Input: part model. Units: mm. Frame: model coordinates. A direction names the side the tool comes from. Coordinates: 2 decimals unless noted, no trailing zeros. Write each loop counter-clockwise with the first axis right and the second up, starting at its lowest first coordinate (ties: lowest second). Pieces come first, ordered by that corner, then holes. Notation, with made-up numbers: (27, 71.5) - (59, 71.5) arc R11 ccw to (59, 79.5) - close; hole circle Ø9 at (-18, 58.25). An arc over 180 degrees is marked (long way). Put each result on its own line as item: value. Start each with the question number.
1. Pull-direction query (Y, two-part tool) for faces 4 (the cylindrical face through (-715.32, 1615.44, -223.05)), 5 (the cylindrical face through (-652.31, 1811.02, -88.74)), 6 (the flat face through (-678, 1443, -180)); classes: released by +Y, released by -Y, zero draft, split by the parting line, or undercut.
2. Cut plane C-C, the plane x = -686. Return loops of the section in (y, z), and give its area (3 significant figures).
3. Cut plane A-A, the plane y = 1465. Return loops of the section in (x, z).
4. Access query for faces 1 (the cylindrical face through (-791.677, 1870.362, -250.236)), 2 (the flat face through (-678, 1443, -330)), 3 (the cylindrical face through (-625.073, 1799.298, -258.88)). Directions: +Z, -Z, +X, -X, +Y, -Y. A direction counts if a zero-diameter tool reaches every point of the face in a straight line with its end or side. Return the directions, or none.
5. Cut plane B-B, the plane z = -314. Return loops of the section in (x, y), and give its area (3 significant figures).
6. Line query: line 1 (Y direction, x = -700, z = -309.5); line 2 (Y direction, x = -700, z = -237); line 3 (Z direction, x = -730.5, y = 1462.5). Output: solid intervals per line, ascending.
7. Cut plane D-D, the plane y = 1796. Return loops of the section in (x, z), and give its area (3 significant figures).
8. Pin query (flat end, axial travel): pin 1 (1 mm diameter, centred on x = -741.5, z = -78, fed in from -Y); pin 2 (1 mm diameter, centred on x = -722.5, y = 1699.5, fed in from -Z); pin 3 (8 mm diameter, centred on x = -757, z = -238.5, fed in from -Y); pin 4 (1.5 mm diameter, centred on y = 1483, z = -177.5, fed in from -X). Return the tip coordinate at first contact, or that it passes through.
from build123d import *

# Parameters (mm, degrees)
SKETCH1_R           = 50
BOSS_EXTRUDE1_DEPTH = 180
SKETCH2_R           = 75
BOSS_EXTRUDE2_DEPTH = 160
SKETCH3_R           = 75
BOSS_EXTRUDE3_DEPTH = 128.18
SKETCH4_R           = 40
BOSS_EXTRUDE4_DEPTH = 300
SKETCH5_R           = 50
SKETCH5_R_2         = 30
BOSS_EXTRUDE5_DEPTH = 150


with BuildPart() as part:
    # Sketch1 → Boss-Extrude1 (new body)
    with BuildSketch(Plane.XY):
        with Locations((-700, 1796)):
            Circle(SKETCH1_R)
    extrude(amount=-BOSS_EXTRUDE1_DEPTH)

    # Sketch2 → Boss-Extrude2 (add)
    with BuildSketch(Plane(origin=(0, 0, -180), x_dir=(-1, 0, 0), z_dir=(0, 0, -1))):
        with Locations((700, 1796)):
            Circle(SKETCH2_R)
    extrude(amount=BOSS_EXTRUDE2_DEPTH)

    # Sketch3 → Boss-Extrude3 (add)
    with BuildSketch(Plane(origin=(-700, 0, 0), x_dir=(0, 0, -1), z_dir=(1, 0, 0))):
        with Locations((260, 1796)):
            Circle(SKETCH3_R)
    extrude(amount=-BOSS_EXTRUDE3_DEPTH)

    # Sketch4 → Boss-Extrude4 (add)
    with BuildSketch(Plane(origin=(0, 1795, 0), x_dir=(-1, 0, 0), z_dir=(0, 1, 0))):
        with Locations(Location((700, -260, 0), (0, 0, 90))):
            Circle(SKETCH4_R)
    extrude(amount=-BOSS_EXTRUDE4_DEPTH)

    # Sketch5 → Boss-Extrude5 (add)
    with BuildSketch(Plane.XY.offset(-180)):
        with Locations((-700, 1465)):
            Circle(SKETCH5_R)
        with Locations((-700, 1465)):
            Circle(SKETCH5_R_2, mode=Mode.SUBTRACT)
    extrude(amount=-BOSS_EXTRUDE5_DEPTH)


solid = part.part
Report:
1. face 4: undercut
1. face 5: split by the parting line
1. face 6: zero draft
2. outline: (1417, -330) - (1438.47, -330) - (1438.47, -180) - (1417, -180) - close; (1491.53, -330) - (1513, -330) - (1513, -297.47) - (1722.32, -297.47) - (1722.32, -340) - (1869.68, -340) - (1869.68, -180) - (1844, -180) - (1844, 0) - (1748, 0) - (1748, -180) - (1722.32, -180) - (1722.32, -222.53) - (1513, -222.53) - (1513, -180) - (1491.53, -180) - close
2. area: 63,000 mm^2
3. outline: (-750, -330) - (-730, -330) - (-730, -180) - (-750, -180) - close; (-670, -330) - (-650, -330) - (-650, -180) - (-670, -180) - close
4. face 1: -X
4. face 2: -Z, +X, -X, -Y
4. face 3: none
5. outline: (-828.18, 1743.95) - (-754, 1743.95) arc R75 ccw (long way) to (-754, 1848.05) - (-828.18, 1848.05) - close; circle Ø100 at (-700, 1465); hole circle Ø60 at (-700, 1465)
5. area: 28,900 mm^2
6. line 1: y = 1415 to 1435, 1495 to 1515, 1721 to 1871
6. line 2: y = 1415 to 1435, 1495 to 1871
6. line 3: z = -330 to -180
7. outline: (-828.18, -335) - (-775, -335) - (-775, -340) - (-625, -340) - (-625, -180) - (-650, -180) - (-650, 0) - (-750, 0) - (-750, -180) - (-775, -180) - (-775, -185) - (-828.18, -185) - close
7. area: 50,000 mm^2
8. pin 1: stops at y = 1767.38
8. pin 2: stops at z = -293.41
8. pin 3: stops at y = 1723.07
8. pin 4: passes through
